The model under review builds one solid part; all positions refer to its coordinate system, in mm. Round coordinates to 2 decimals unless told otherwise and drop trailing zeros. Order: outer loops, then holes, each group sorted by start corner. A loop starts at its lowest first (then second) coordinate and runs counter-clockwise, first axis right, second up. Notation, with made-up numbers: M -18,38.25 L 41,38.25 A34 ccw 41,70.25 Z; hole C 2.5,73 d11. An arc over 180 degrees is marked long. Answer as CSV lines item,"result". Start each with the question number.
from build123d import *

# Parameters (mm, degrees)
SKETCH1_R           = 20
BOSS_EXTRUDE1_DEPTH = 10


with BuildPart() as part:
    # Sketch1 → Boss-Extrude1 (new body)
    with BuildSketch(Plane.XY):
        with BuildLine():
            Line((56.23475383, -20.920144878), (75.334884287, -31.947610338))
            ThreePointArc((75.334884287, -31.947610338), (120.810543828, -69.75), (65.334884287, -49.268118414))
            Line((65.334884287, -49.268118414), (46.23475383, -38.240652953))
            ThreePointArc((46.23475383, -38.240652953), (30, -51.961524227), (10, -59.160797831))
            Line((10, -59.160797831), (10, -81.215728753))
            ThreePointArc((10, -81.215728753), (0, -139.5), (-10, -81.215728753))
            Line((-10, -81.215728753), (-10, -59.160797831))
            ThreePointArc((-10, -59.160797831), (-30, -51.961524227), (-46.23475383, -38.240652953))
            Line((-46.23475383, -38.240652953), (-65.334884287, -49.268118414))
            ThreePointArc((-65.334884287, -49.268118414), (-120.810543828, -69.75), (-75.334884287, -31.947610338))
            Line((-75.334884287, -31.947610338), (-56.23475383, -20.920144878))
            ThreePointArc((-56.23475383, -20.920144878), (-60, 0), (-56.23475383, 20.920144878))
            Line((-56.23475383, 20.920144878), (-75.334884287, 31.947610338))
            ThreePointArc((-75.334884287, 31.947610338), (-120.810543828, 69.75), (-65.334884287, 49.268118414))
            Line((-65.334884287, 49.268118414), (-46.23475383, 38.240652953))
            ThreePointArc((-46.23475383, 38.240652953), (-30, 51.961524227), (-10, 59.160797831))
            Line((-10, 59.160797831), (-10, 81.215728753))
            ThreePointArc((-10, 81.215728753), (0, 139.5), (10, 81.215728753))
            Line((10, 81.215728753), (10, 59.160797831))
            ThreePointArc((10, 59.160797831), (30, 51.961524227), (46.23475383, 38.240652953))
            Line((46.23475383, 38.240652953), (65.334884287, 49.268118414))
            ThreePointArc((65.334884287, 49.268118414), (120.810543828, 69.75), (75.334884287, 31.947610338))
            Line((75.334884287, 31.947610338), (56.23475383, 20.920144878))
            ThreePointArc((56.23475383, 20.920144878), (60, 0), (56.23475383, -20.920144878))
        make_face()
        with Locations((94.829781714, 54.75)):
            Circle(SKETCH1_R, mode=Mode.SUBTRACT)
        with Locations((94.829781714, -54.75)):
            Circle(SKETCH1_R, mode=Mode.SUBTRACT)
        with Locations((0, -109.5)):
            Circle(SKETCH1_R, mode=Mode.SUBTRACT)
        with Locations((-94.829781714, -54.75)):
            Circle(SKETCH1_R, mode=Mode.SUBTRACT)
        with Locations((-94.829781714, 54.75)):
            Circle(SKETCH1_R, mode=Mode.SUBTRACT)
        with Locations((0, 109.5)):
            Circle(SKETCH1_R, mode=Mode.SUBTRACT)
        with BuildLine():
            ThreePointArc((25.529394822, 11.5), (0, 28), (-25.529394822, 11.5))
            Line((-25.529394822, 11.5), (-35, 11.5))
            Line((-35, 11.5), (-35, -11.5))
            Line((-35, -11.5), (-25.529394822, -11.5))
            ThreePointArc((-25.529394822, -11.5), (0, -28), (25.529394822, -11.5))
            Line((25.529394822, -11.5), (35, -11.5))
            Line((35, -11.5), (35, 11.5))
            Line((35, 11.5), (25.529394822, 11.5))
        make_face(mode=Mode.SUBTRACT)
    extrude(amount=BOSS_EXTRUDE1_DEPTH)


solid = part.part
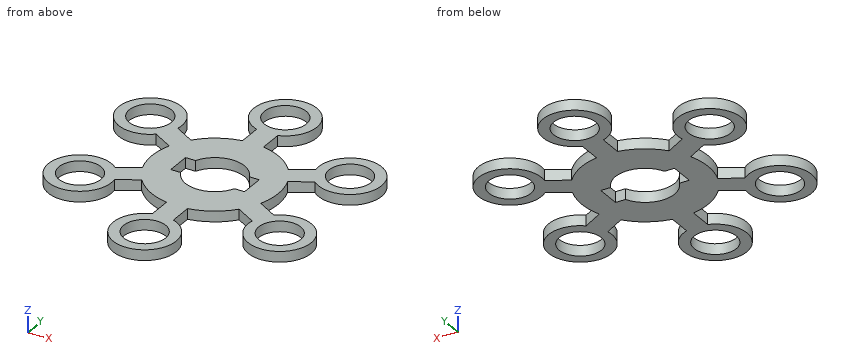
Item 1: For pin 1 (3 mm diameter, centred on y = 74, z = 3.5, fed in from -X); pin 2 (5 mm diameter, centred on y = -73, z = 5.5, fed in from +X); pin 3 (6 mm diameter, centred on x = -86, z = 2, fed in from +Y); pin 4 (5 mm diameter, centred on x = 20, y = -60.5, fed in from -Z), all flat-tipped, find the tip position at first contact; note any pin that passes through.
Item 2: Consider section C-C (y = 54.75). State the section outline as (x, z) points, and give its area (3 significant figures).
Item 3: Wall thickness on probe 1 along X at (y, z) = (40.5, 3.75); probe 2 along X at (y, z) = (-62, 8.5); probe 3 along Y at (x, z) = (-17, 5.5): over which ranges is each line inside the solid? List them lowest first. Write a range as [from, to].
Item 4: Consider section D-D (z = 4.5). State how many separate pieces and enclosed holes the cut face has, and give its area (3 significant figures).
Item 5: Consider section B-B (x = 0). State the section outline as (y, z) points, and give its area (3 significant figures).
Item 6: Consider section A-A (y = -109.5). State the section outline as (x, z) points.
Reported:
1,pin 1,"stops at x = -119.02"
1,pin 2,"stops at x = 120.36"
1,pin 3,"stops at y = 84.18"
1,pin 4,"passes through"
2,outline,"M -124.83,0 L -114.83,0 L -114.83,10 L -124.83,10 Z; M -74.83,0 L -64.83,0 L -64.83,10 L -74.83,10 Z; M -24.54,0 L 24.54,0 L 24.54,10 L -24.54,10 Z; M 64.83,0 L 74.83,0 L 74.83,10 L 64.83,10 Z; M 114.83,0 L 124.83,0 L 124.83,10 L 114.83,10 Z"
2,area,"891 mm²"
3,probe 1,"x = [-121.23, -108.86], [-80.8, -50.15], [-44.27, 44.27], [50.15, 80.8], [108.86, 121.23]"
3,probe 2,"x = [-123.94, -113.47], [-76.19, -65.72], [-10, 10], [65.72, 76.19], [113.47, 123.94]"
3,probe 3,"y = [-134.22, -120.04], [-98.96, -84.78], [-57.54, -22.25], [22.25, 57.54], [84.78, 98.96], [120.04, 134.22]"
4,separate pieces,"1"
4,enclosed holes,"7"
4,area,"20,400 mm²"
5,outline,"M -139.5,0 L -129.5,0 L -129.5,10 L -139.5,10 Z; M -89.5,0 L -28,0 L -28,10 L -89.5,10 Z; M 28,0 L 89.5,0 L 89.5,10 L 28,10 Z; M 129.5,0 L 139.5,0 L 139.5,10 L 129.5,10 Z"
5,area,"1,430 mm²"
6,outline,"M -30,0 L -20,0 L -20,10 L -30,10 Z; M 20,0 L 30,0 L 30,10 L 20,10 Z"
